```python
from build123d import *

# Parameters (mm, degrees)
SKETCH1_R           = 2.5
SKETCH1_R_2         = 19
SKETCH1_R_3         = 22.5
SKETCH1_R_4         = 2
BOSS_EXTRUDE1_DEPTH = 5


with BuildPart() as part:
    # Sketch1 → Boss-Extrude1 (new body)
    with BuildSketch(Plane.XY):
        with BuildLine():
            Line((30.000692042, 92.545526446), (235.000692042, 92.545526446))
            ThreePointArc((235.000692042, 92.545526446), (238.536225947, 91.081060352), (240.000692042, 87.545526446))
            Line((240.000692042, 87.545526446), (240.000692042, -52.454473554))
            ThreePointArc((240.000692042, -52.454473554), (238.536225947, -55.99000746), (235.000692042, -57.454473554))
            Line((235.000692042, -57.454473554), (30.000692042, -57.454473554))
            ThreePointArc((30.000692042, -57.454473554), (-44.999307958, 17.545526446), (30.000692042, 92.545526446))
        make_face()
        with Locations((-34.999307958, 17.545526446)):
            Circle(SKETCH1_R, mode=Mode.SUBTRACT)
        with Locations((30.000692042, -47.454473554)):
            Circle(SKETCH1_R, mode=Mode.SUBTRACT)
        with Locations((30.000692042, 82.545526446)):
            Circle(SKETCH1_R, mode=Mode.SUBTRACT)
        with Locations((230.000692042, -47.454473554)):
            Circle(SKETCH1_R, mode=Mode.SUBTRACT)
        with Locations((230.000692042, 82.545526446)):
            Circle(SKETCH1_R, mode=Mode.SUBTRACT)
        with Locations((130.000692042, 82.545526446)):
            Circle(SKETCH1_R, mode=Mode.SUBTRACT)
        with Locations((130.000692042, -47.454473554)):
            Circle(SKETCH1_R, mode=Mode.SUBTRACT)
        with Locations((199.000692042, 17.545526446)):
            Circle(SKETCH1_R_2, mode=Mode.SUBTRACT)
        with Locations((30.000692042, 17.545526446)):
            Circle(SKETCH1_R_3, mode=Mode.SUBTRACT)
        with Locations((61.815692042, 49.360526446)):
            Circle(SKETCH1_R_4, mode=Mode.SUBTRACT)
        with Locations((61.815692042, -14.269473554)):
            Circle(SKETCH1_R_4, mode=Mode.SUBTRACT)
        with Locations((-1.814307958, -14.269473554)):
            Circle(SKETCH1_R_4, mode=Mode.SUBTRACT)
        with Locations((-1.814307958, 49.360526446)):
            Circle(SKETCH1_R_4, mode=Mode.SUBTRACT)
        with BuildLine():
            Line((77.500692042, 19.545526446), (82.500692042, 19.545526446))
            ThreePointArc((82.500692042, 19.545526446), (84.500692042, 17.545526446), (82.500692042, 15.545526446))
            Line((82.500692042, 15.545526446), (77.500692042, 15.545526446))
            ThreePointArc((77.500692042, 15.545526446), (75.500692042, 17.545526446), (77.500692042, 19.545526446))
        make_face(mode=Mode.SUBTRACT)
        with BuildLine():
            Line((101.500692042, 19.545526446), (96.500692042, 19.545526446))
            ThreePointArc((96.500692042, 19.545526446), (94.500692042, 17.545526446), (96.500692042, 15.545526446))
            Line((96.500692042, 15.545526446), (101.500692042, 15.545526446))
            ThreePointArc((101.500692042, 15.545526446), (103.500692042, 17.545526446), (101.500692042, 19.545526446))
        make_face(mode=Mode.SUBTRACT)
    extrude(amount=BOSS_EXTRUDE1_DEPTH)


solid = part.part
```
CAD build for the part. Positions are in the model's coordinates, mm. A direction names the side the tool comes from. Round coordinates to 2 decimals unless told otherwise and drop trailing zeros. Order: outer loops, then holes, each group sorted by start corner. A loop starts at its lowest first (then second) coordinate and runs counter-clockwise, first axis right, second up.
Item 1: Saw through at D-D on y = 4. Write the cut outline in (x, z).
Item 2: Mould opens along Y. For faces 1 (the face through (99, 19.546, 2)), 2 (the face through (240.001, 19, 2)), 3 (the face through (-44.98, 15.9, 2.46)) say: pulls with the +Y half, pulls with the -Y half, needs draft (parallel to the pull), parting line crosses it, or undercut.
Item 3: Saw through at B-B on z = 1.65. State how many separate pieces and enclosed holes the cut face has, then the cut area to 3 significant figures.
Item 4: Saw through at A-A on y = 30. Write the cut outline in (x, z).
Item 5: Probe line 1 along Y through (x, z) = (62, 3.7); line 2 along Y through (x, z) = (78, 2.45); line 3 along X through (y, z) = (21, 2.4). List the from-to ranges inside material, lowest first.
Item 6: Tool access for faces 4 (the face through (238.497, 91.12, 2.465)), 5 (the face through (80, 15.546, 2)): list every direction of +Z, -Z, +X, -X, +Y, -Y with a clear straight run to the whole face (end or side of a thin tool).
Item 7: Pin check, flat tip, straight feed: pin 1 (4 mm diameter, centred on x = -35, y = 17.55, fed in from -Z). Stop position of the tip, or through.
Item 8: Saw through at C-C on x = 19.5. Write the cut outline in (y, z), then the cut area to 3 significant figures.
Reported:
1. outline: (-43.77, 0) - (12.03, 0) - (12.03, 5) - (-43.77, 5) - close; (47.97, 0) - (185.68, 0) - (185.68, 5) - (47.97, 5) - close; (212.32, 0) - (240, 0) - (240, 5) - (212.32, 5) - close
2. face 1: undercut
2. face 2: needs draft
2. face 3: parting line crosses it
3. separate pieces: 1
3. enclosed holes: 15
3. area: 37,300 mm2
4. outline: (-43.96, 0) - (11.26, 0) - (11.26, 5) - (-43.96, 5) - close; (48.74, 0) - (184.65, 0) - (184.65, 5) - (48.74, 5) - close; (213.35, 0) - (240, 0) - (240, 5) - (213.35, 5) - close
5. line 1: y = -57.45 to -16.26, -12.28 to 47.37, 51.35 to 92.55
5. line 2: y = -57.45 to 15.55, 19.55 to 92.55
5. line 3: x = -44.92 to 7.77, 52.23 to 180.32, 217.68 to 240
6. face 4: +Z, -Z, +X, +Y
6. face 5: +Z, -Z
7. pin 1: passes through
8. outline: (-56.72, 0) - (-2.35, 0) - (-2.35, 5) - (-56.72, 5) - close; (37.44, 0) - (91.81, 0) - (91.81, 5) - (37.44, 5) - close
8. area: 544 mm2
